```python
from build123d import *

# Parameters (mm, degrees)
BOSS_EXTRUDE1_DEPTH = 1.5
SKETCH12_W          = 29
SKETCH12_H          = 12
BOSS_EXTRUDE2_DEPTH = 6


with BuildPart() as part:
    # Sketch1 → Boss-Extrude1 (new body)
    with BuildSketch(Plane.XY):
        Polygon((0, 6), (0.314446676, 0), (1.497941481, 0), (1.657221927, 3.039251967), (2.042586863, 3.65596478), (2.769801294, 3.65596478), (3.155166229, 3.039251967), (3.314446676, 0), (4.497941481, 0), (4.657221927, 3.039251967), (5.042586863, 3.65596478), (5.769801294, 3.65596478), (6.155166229, 3.039251967), (6.314446676, 0), (7.497941481, 0), (7.657221927, 3.039251967), (8.042586863, 3.65596478), (8.769801294, 3.65596478), (9.155166229, 3.039251967), (9.314446676, 0), (10.497941481, 0), (10.657221927, 3.039251967), (11.042586863, 3.65596478), (11.769801294, 3.65596478), (12.155166229, 3.039251967), (12.314446676, 0), (13.497941481, 0), (13.657221927, 3.039251967), (14.042586863, 3.65596478), (16.269801294, 3.65596478), (16.655166229, 3.039251967), (16.814446676, 0), (17.997941481, 0), (18.312388157, 6), (24.156194078, 6), (24.156194078, 20.5), (-5.843805922, 20.5), (-5.843805922, 6), align=None)
    extrude(amount=BOSS_EXTRUDE1_DEPTH)

    # Sketch12 → Boss-Extrude2 (add)
    with BuildSketch(Plane.XY):
        with Locations((9.156194078, 14)):
            Rectangle(SKETCH12_W, SKETCH12_H)
    extrude(amount=-BOSS_EXTRUDE2_DEPTH)


solid = part.part
```
Geometry check sheet. Reference: the model listing, model coordinates, mm. A direction names the side the tool comes from. Coordinates: 2 decimals unless noted, no trailing zeros. Write each loop counter-clockwise with the first axis right and the second up, starting at its lowest first coordinate (ties: lowest second). Pieces come first, ordered by that corner, then holes. Notation, with made-up numbers: (73, 17.5) -> (131, 17.5) arc R9 ccw to (131, 24.5) -> close; hole circle Ø7 at (69.5, 55.5). An arc over 180 degrees is marked (long way). Use CSV: the item, a comma, the result in double quotes. Start each with the question number.
Item 1: Mould release check, pull along X, two halves, no side actions. Record for faces 4 (the flat face through (24.156, 13, 1)), 5 (the flat face through (7, 7, 0)), 6 (the flat face through (0.155, 3.042, 0.74)), 7 (the flat face through (16.734, 1.541, 0.74)): released by +X, released by -X, zero draft, split by the parting line, or undercut.
Item 2: Thickness scan on line 1 (Y direction, x = 12.25, z = -2.25); line 2 (Z direction, x = 6, y = 4.75); line 3 (Y direction, x = 5.5, z = 0.25). Record the ranges inside material, lowest first.
Item 3: Cross-section at D-D, the plane z = -2. Record the cut outline in (x, y).
Item 4: Cross-section at C-C, the plane y = 12. Record the cut outline in (x, z), plus the area to 3 significant figures.
Item 5: Depth check by flat-ended pin: pin 1 Ø4 at (x, z) = (15.5, -5) entering from -Y; pin 2 Ø2 at (y, z) = (14, -4) entering from +X; pin 3 Ø2 at (x, z) = (0, -3) entering from +Y. Enter the tip coordinate at first touch or a pass-through.
Item 6: Cross-section at B-B, the plane x = 15.25. Record the cut outline in (y, z).
Item 7: Cross-section at A-A, the plane y = 1.75. Record the cut outline in (x, z).
Item 8: Set-up check for faces 1 (the flat face through (9, 8, -3)), 2 (the flat face through (21, 6, 1)), 3 (the flat face through (12.234, 1.541, 0.74)): record each of +Z, -Z, +X, -X, +Y, -Y from which the full face is reachable in a straight line by a thin tool's end or side.
Answers:
1,face 4,"released by +X"
1,face 5,"zero draft"
1,face 6,"released by -X"
1,face 7,"undercut"
2,line 1,"8 to 20"
2,line 2,"0 to 1.5"
2,line 3,"3.66 to 20.5"
3,outline,"(-5.34, 8) -> (23.66, 8) -> (23.66, 20) -> (-5.34, 20) -> close"
4,outline,"(-5.84, 0) -> (-5.34, 0) -> (-5.34, -6) -> (23.66, -6) -> (23.66, 0) -> (24.16, 0) -> (24.16, 1.5) -> (-5.84, 1.5) -> close"
4,area,"219 mm^2"
5,pin 1,"y = 8"
5,pin 2,"x = 23.66"
5,pin 3,"y = 20"
6,outline,"(3.66, 0) -> (8, 0) -> (8, -6) -> (20, -6) -> (20, 0) -> (20.5, 0) -> (20.5, 1.5) -> (3.66, 1.5) -> close"
7,outline,"(0.22, 0) -> (1.59, 0) -> (1.59, 1.5) -> (0.22, 1.5) -> close; (3.22, 0) -> (4.59, 0) -> (4.59, 1.5) -> (3.22, 1.5) -> close; (6.22, 0) -> (7.59, 0) -> (7.59, 1.5) -> (6.22, 1.5) -> close; (9.22, 0) -> (10.59, 0) -> (10.59, 1.5) -> (9.22, 1.5) -> close; (12.22, 0) -> (13.59, 0) -> (13.59, 1.5) -> (12.22, 1.5) -> close; (16.72, 0) -> (18.09, 0) -> (18.09, 1.5) -> (16.72, 1.5) -> close"
8,face 1,"-Z, +X, -X, -Y"
8,face 2,"+Z, -Z, +X, -Y"
8,face 3,"+Z, -Z, -Y"
